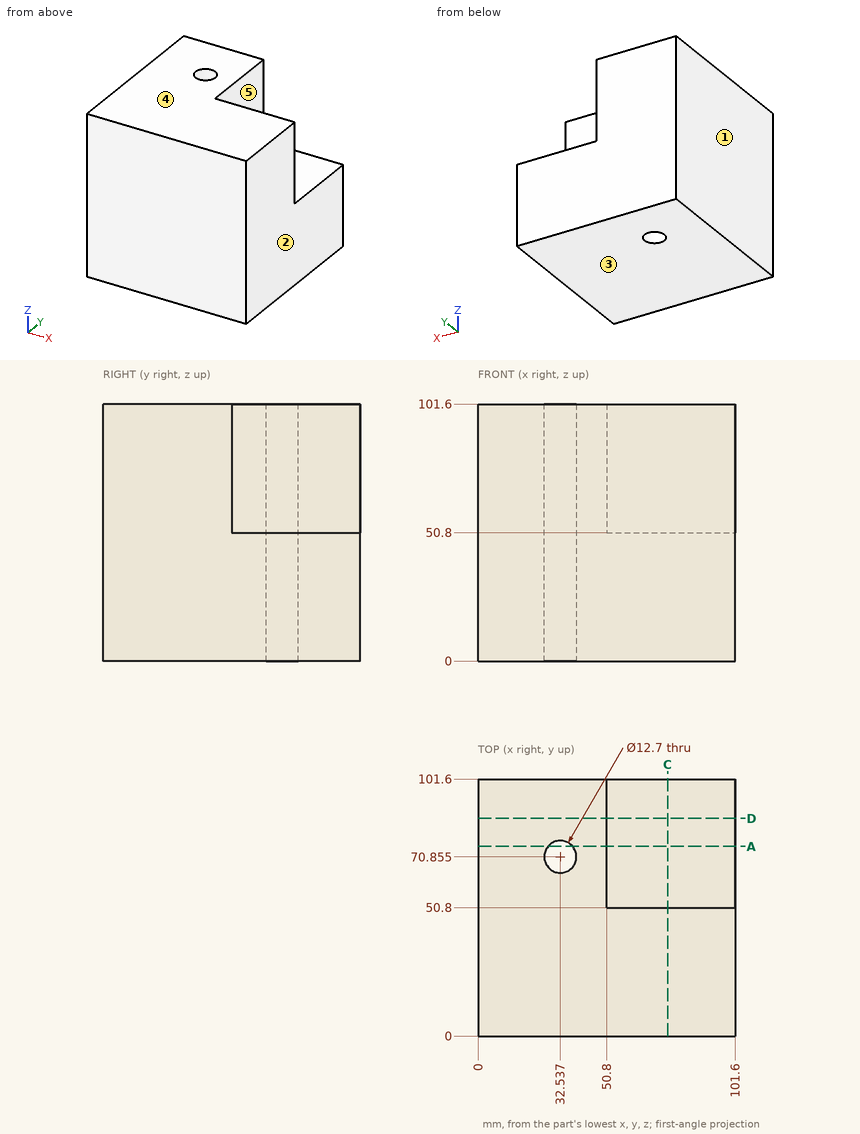
Verification items for this drawing (mm, ordinates from the low corner). A direction names the side the tool comes from. Coordinates: 2 decimals unless noted, no trailing zeros. Write each loop counter-clockwise with the first axis right and the second up, starting at its lowest first coordinate (ties: lowest second). Pieces come first, ordered by that corner, then holes. Notation, with made-up numbers: M -39.5,5.25 L -20.5,5.25 A8 ccw -20.5,18.25 Z; hole C 60.25,-5 d4. An arc over 180 degrees is marked long. Answer as a JSON object with one key per item and string values.
1. Draft check along X on the marked faces 1, 2 and 3. Enter one of: released by +X, released by -X, zero draft, split by the parting line, or undercut.
Answers below:
{"face 1": "released by -X", "face 2": "released by +X", "face 3": "zero draft"}
2. Section check C-C, the plane x = 75. Enter the section's corners in (y, z).
Answers below:
{"outline": "M 0,0 L 101.6,0 L 101.6,50.8 L 50.8,50.8 L 50.8,101.6 L 0,101.6 Z"}
3. Tool access check on the marked faces 4 and 5. Record the directions out of +Z, -Z, +X, -X, +Y, -Y that give a thin tool (end or side, any length) a straight path to the whole face; none if there is none.
Answers below:
{"face 4": "+Z, +X, -X, +Y, -Y", "face 5": "+Z, +X, +Y"}
4. Go/stop test with flat-tipped pins: pin 1 Ø15 at (x, y) = (82, 81.5) entering from +Z; pin 2 Ø3 at (x, z) = (65, 65) entering from +Y; pin 3 Ø15 at (y, z) = (73.5, 68) entering from +X. Record where each tip stops, or that it passes through.
Answers below:
{"pin 1": "stops at z = 50.8", "pin 2": "stops at y = 50.8", "pin 3": "stops at x = 50.8"}
5. Section check A-A, the plane y = 75. Enter the section's corners in (x, z).
Answers below:
{"outline": "M 0,0 L 27.73,0 L 27.73,101.6 L 0,101.6 Z; M 37.35,0 L 101.6,0 L 101.6,50.8 L 50.8,50.8 L 50.8,101.6 L 37.35,101.6 Z"}
6. Scan lines: L1, parallel to X at y = 95, z = 79; L2, parallel to X at y = 71.5, z = 8; L3, parallel to X at y = 70.5, z = 89. Record each from-to range of solid material in increasing order.
Answers below:
{"L1": "x = 0 to 50.8", "L2": "x = 0 to 26.22, 38.85 to 101.6", "L3": "x = 0 to 26.2, 38.88 to 50.8"}
